Source: CAD feature listing. Evaluate the final solid. Frame: model axes, mm. A direction names the side the tool comes from. Round coordinates to 2 decimals unless told otherwise and drop trailing zeros. Order: outer loops, then holes, each group sorted by start corner. A loop starts at its lowest first (then second) coordinate and runs counter-clockwise, first axis right, second up. Notation, with made-up numbers: (-5.75, 51.25) - (28.25, 51.25) arc R25 cw to (28.25, 86.25) - close; hole circle Ø8 at (-36, 52). An arc over 180 degrees is marked (long way). Put each result on its own line as item: value. Start each with the question number.
1) Section A-A on y = 8. Output: boundary loops of the cut face in (x, z).
2) Line query: probe 1 along Z at (x, y) = (5, 29); probe 2 along Y at (x, z) = (2.25, 3.75); probe 3 along Y at (x, z) = (2.25, -1.5) (3 decimals). Output: solid intervals per line, ascending. Write a range as [from, to].
3) Access query for faces 1 (the face through (5.3, 21.55, 1.67)), 2 (the face through (-2, 0, -2)). Directions: +Z, -Z, +X, -X, +Y, -Y. A direction counts if a zero-diameter tool reaches every point of the face in a straight line with its end or side. Return the directions, or none.
4) Contact query for flat-ended pins moving along their axis: P1, Ø7.5, axis at x = 1, z = 1, coming from the +Y side; P2, Ø2, axis at y = 4.5, z = 3.5, coming from the -X side; P3, Ø5, axis at x = 0, z = 0, coming from the -Y side. Output: stop coordinate, or through.
5) Mould query, pull axis X, two halves, no side actions, for faces 3 (the face through (0, 3.175, 3)), 4 (the face through (-2, 10.319, -4)), 5 (the face through (-2, 32.544, -6)), 6 (the face through (6.853, 3.618, 2.158)). Classes: +X half, -X half, draft (parallel to the pull), parting line (faces both ways), or undercut.
```python
from build123d import *

# Parameters (mm, degrees)
FILLET2_R     = 6.35
FILLET3_R     = 1.5875
FILLET1_R     = 0.79375
CHAMFER1_SIZE = 0.254


with BuildPart() as part:
    # Sketch1 → Revolve1 (revolve)
    with BuildSketch(Plane.XY):
        Polygon((8.73125, 32.54375), (5.55625, 32.54375), (5.55625, 10.31875), (3.96875, 10.31875), (3.96875, 3.175), (2.38125, 3.175), (2.38125, 0), (6.35, 0), (8.73125, 10.31875), align=None)
    revolve(axis=Axis((0, 4.297998533, 0), (0, -1, 0)))

    # Fillet2
    fillet2_edges = [part.edges().sort_by_distance(p)[0] for p in [
        (-8.73125, 10.31875, 0),
    ]]
    fillet(fillet2_edges, radius=FILLET2_R)

    # Fillet3
    fillet3_edges = [part.edges().sort_by_distance(p)[0] for p in [
        (-6.35, 0, 0),
    ]]
    fillet(fillet3_edges, radius=FILLET3_R)

    # Fillet1
    fillet1_edges = [part.edges().sort_by_distance(p)[0] for p in [
        (-5.55625, 10.31875, 0),
        (-3.96875, 3.175, 0),
    ]]
    fillet(fillet1_edges, radius=FILLET1_R)

    # Chamfer1
    chamfer1_edges = [part.edges().sort_by_distance(p)[0] for p in [
        (-2.38125, 0, 0),
        (-8.73125, 32.54375, 0),
        (-5.55625, 32.54375, 0),
        (-3.96875, 10.31875, 0),
        (-2.38125, 3.175, 0),
    ]]
    chamfer(chamfer1_edges, length=CHAMFER1_SIZE)


solid = part.part
```
Answer sheet:
1. outline: circle Ø16.39 at (0, 0); hole circle Ø7.94 at (0, 0)
2. probe 1: [-7.16, -2.42], [2.42, 7.16]
2. probe 2: [0, 10.32]
2. probe 3: [0, 3.175]
3. face 1: +Y
3. face 2: +Z, -Z, +X, -X, -Y
4. P1: y = 10.43
4. P2: x = -7.03
4. P3: y = 0.14
5. face 3: undercut
5. face 4: undercut
5. face 5: draft
5. face 6: parting line
